from build123d import *

# Parameters (mm, degrees)
F0_R     = 12.5
F1_DEPTH = 0.7
F2_R     = 0.4
F2_W     = 0.8
F2_H     = 0.8
F2_W_2   = 10
F2_H_2   = 0.4
F3_DEPTH = 5.7


with BuildPart() as f1:
    # F0 (on Top) → F1 (new body)
    with BuildSketch(Plane.XY):
        Circle(F0_R)
    extrude(amount=F1_DEPTH)

    # F2 (on Top) → F3 (join)
    with BuildSketch(Plane.XY):
        with Locations((-1.5, 1.5)):
            Circle(F2_R)
        with Locations((-1.5, -1.5)):
            Circle(F2_R)
        with Locations((1.5, -1.5)):
            Circle(F2_R)
        with Locations((1.5, 1.5)):
            Circle(F2_R)
        with Locations((2.914214, -2.914214)):
            Circle(F2_R)
        with Locations((5.742641, 5.742641)):
            Circle(F2_R)
        with Locations((-5.035534, 5.035534)):
            Circle(F2_R)
        with Locations((-4.328427, -4.328427)):
            Circle(F2_R)
        with Locations((0.031655, 9.595732)):
            Rectangle(F2_W, F2_H)
        Polygon((-8.801591, 0.723574), (-9.757094, 0.428594), (-9.757094, -0.571406), (-8.774174, -0.755441), (-8.114989, -0.00346), align=None)
        Polygon((9.806349, -0.655786), (9.306349, 0.21024), (8.806349, -0.655786), align=None)
        with Locations((0.377344, -8.348521)):
            Rectangle(F2_W_2, F2_H_2)
    extrude(amount=F3_DEPTH)


solid = f1.part
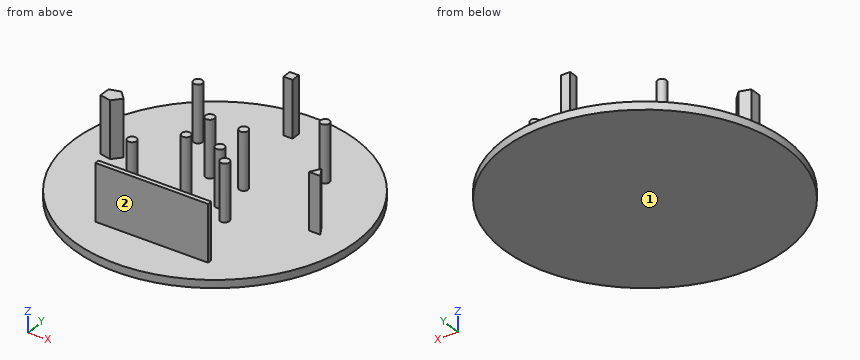
Input: part model. Units: mm. Frame: model coordinates. Face numbers are marked on the shaded views. A direction names the side the tool comes from. Give positions to 0.01 mm unless a question says otherwise; leave off trailing zeros. Order: outer loops, then holes, each group sorted by start corner. A loop starts at its lowest first (then second) coordinate and runs counter-clockwise, first axis right, second up. Notation, with made-up numbers: (47.25, 51.25) - (66.25, 51.25) arc R29 ccw to (66.25, 78.25) - close; hole circle Ø2 at (18, 66). An arc over 180 degrees is marked (long way). Answer as a JSON object with one key per item and string values. Group by question number.
Q1. Set-up query: the marked faces 1 and 2. Return all of +Z, -Z, +X, -X, +Y, -Y with unobstructed straight access to the full face (end or side cutting, diameter ignored); none if empty.
Q2. Cut plane C-C, the plane y = 1.5. Output: boundary loops of the cut face in (x, z), then the cut area to 3 significant figures.
Q3. Cut plane D-D, the plane y = 10.5. Output: boundary loops of the cut face in (x, z), then the cut area to 3 significant figures.
Q4. Cut plane B-B, the plane x = 0. Output: boundary loops of the cut face in (y, z), then the cut area to 3 significant figures.
Q5. Cut plane A-A, the plane z = 1.4. Count the separate pieces of the cut face and the enclosed holes in it, then the cut area to 3 significant figures.
Q6. First-contact query: pin 1 Ø1.5 at (y, z) = (3.5, 1) entering from +X; pin 2 Ø2 at (x, z) = (9, 5) entering from +Y; pin 3 Ø1.1 at (y, z) = (0, 4.5) entering from -X. Flat tips, straight axial feed; report the tip coordinate or a pass-through.
Q7. Line query: probe 1 along Z at (x, y) = (2.25, 7); probe 2 along Y at (x, z) = (-2, 1.2); probe 3 along Y at (x, z) = (1.25, 4.9). Output: solid intervals per line, ascending.
Results:
{
 "1": {"face 1": "-Z, +X, -X, +Y, -Y", "face 2": "+Z, +X, -X, -Y"},
 "2": {"outline": "(-12.41, 0) - (12.41, 0) - (12.41, 0.7) - (1.9, 0.7) - (1.9, 5.7) - (1.1, 5.7) - (1.1, 0.7) - (-1.1, 0.7) - (-1.1, 5.7) - (-1.9, 5.7) - (-1.9, 0.7) - (-12.41, 0.7) - close", "area": "25.4 mm^2"},
 "3": {"outline": "(-6.78, 0) - (6.78, 0) - (6.78, 0.7) - (-6.78, 0.7) - close", "area": "9.50 mm^2"},
 "4": {"outline": "(-12.5, 0) - (12.5, 0) - (12.5, 0.7) - (10, 0.7) - (10, 5.7) - (9.2, 5.7) - (9.2, 0.7) - (-8.15, 0.7) - (-8.15, 5.7) - (-8.55, 5.7) - (-8.55, 0.7) - (-12.5, 0.7) - close", "area": "23.5 mm^2"},
 "5": {"separate pieces": "12", "enclosed holes": "0", "area": "10.8 mm^2"},
 "6": {"pin 1": "x = 12.18", "pin 2": "y = 0.21", "pin 3": "x = -9.76"},
 "7": {"probe 1": "0 to 0.7", "probe 2": "-8.55 to -8.15", "probe 3": "-8.55 to -8.15, -1.81 to -1.19, 1.19 to 1.81"}
}
